Autodesk Inventor part; units mm, degrees
ref_plane "YZ Plane" through (0, 0, 0) normal (1, 0, 0) x (0, 1, 0)
ref_plane "XZ Plane" through (0, 0, 0) normal (0, 1, 0) x (-1, 0, 0)
ref_plane "XY Plane" through (0, 0, 0) normal (0, 0, 1) x (1, 0, 0)
sketch "スケッチ1" plane through (0, 0, 0) normal (0, 0, 1) x (1, 0, 0)
  line L0 (0, 55) -> (20, 55)
  line L1 (20, 55) -> (20, 0)
  line L2 (20, 0) -> (0, 0)
  line L3 (0, 0) -> (0, 55)
  dimension "d0" = 20
  dimension "d1" = 55
extrude "押し出し1" add sketch "スケッチ1" along normal blind 10
chamfer "面取り1" distance 7 angle 45 4 edges at (20, 27.5, 10) (0, 27.5, 10) (10, 55, 10) (10, 0, 10)
sketch "スケッチ2" plane through (0, 0, 0) normal (0, 0, -1) x (-1, 0, 0)
  line L0 (0, 0) -> (-20, 0)
  line L1 (0, 55) -> (0, 0)
  line L2 (-20, 55) -> (0, 55)
  line L3 (-20, 0) -> (-20, 55)
  circle A0 centre (-10, 41.25) radius 0.8
  circle A1 centre (-10, 13.75) radius 0.8
  circle A2 centre (-10, 27.5) radius 0.8
  point P0 (-10, 55)
  dimension "d7" = 1.6
  dimension "d8" = 1.6
  dimension "d9" = 1.6
  dimension "d10" = 13.75
  dimension "d11" = 13.75
  dimension "d12" = 13.75
  dimension "d13" = 13.75
extrude "押し出し2" cut sketch "スケッチ2" against normal through all contours A0 | A1 | A2
sketch "スケッチ3" plane through (0, 0, 10) normal (0, 0, 1) x (1, 0, 0)
  circle A0 centre (10, 41.25) radius 0.8
  circle A1 centre (10, 27.5) radius 0.8
  circle A2 centre (10, 13.75) radius 0.8
  circle A3 centre (10, 27.5) radius 0.8
  circle A4 centre (10, 41.25) radius 0.8
  line L0 (7, 7) -> (7, 48)
  line L1 (13, 7) -> (7, 7)
  line L2 (13, 48) -> (13, 7)
  line L3 (7, 48) -> (13, 48)
  circle A5 centre (10, 41.25) radius 2.5
  circle A6 centre (10, 27.5) radius 2.5
  circle A7 centre (10, 13.75) radius 2.5
  point P0 (0, 0)
  dimension "d16" = 5
  dimension "d17" = 5
  dimension "d18" = 5
extrude "押し出し3" cut sketch "スケッチ3" against normal blind 8.5 contours A5 | A6 | A7
equation "\"d10\" = d13"
equation "\"d11\" = d13"
equation "\"d12\" = d13"
properties part number "shield"
Read the model definition and answer for the solid it produces. Units are mm, in the model's axes. A direction names the side the tool comes from. Give positions to 0.01 mm unless a question says otherwise; leave off trailing zeros. Write each loop counter-clockwise with the first axis right and the second up, starting at its lowest first coordinate (ties: lowest second). Pieces come first, ordered by that corner, then holes. Notation, with made-up numbers: (-21, -27.5) -> (23, -27.5) arc R24 cw to (23, -13.5) -> close; hole circle Ø4 at (5.25, -11.75). An arc over 180 degrees is marked (long way). Answer as a JSON object with one key per item and string values. Group by question number.
1) Find section C-C (x = 10). Count the separate pieces of the cut face and the enclosed holes in it, and give its area (3 significant figures).
2) A tool of negligible diameter and unlimited length cuts with its end or side. For faces 4 (the flat face through (9, 14, 1.5)), 5 (the flat face through (10, 3, 6)), from which of +Z, -Z, +X, -X, +Y, -Y can it reach the whole face along a straight path? Write none if from no direction.
3) Find section A-A (y = 27.5). Write down the section's boundary in (x, z), and give its area (3 significant figures).
4) Find section D-D (x = 15.75). Write down the section's boundary in (y, z).
5) Find section B-B (z = 2.25). Write down the section's boundary in (x, y).
6) Consider L1, parallel to Y at x = 10, z = 0.9; L2, parallel to Y at x = 10, z = 5.5; L3, parallel to X at y = 27.5, z = 0.4. Determine where each line is inside the solid, lowest interval first. Write a range as from..to.
7) The mould has two halves that part along Y. Classify faces 1 (the flat face through (20, 28, 1)), 2 (the flat face through (10, 55, 1)), 3 (the cylindrical face through (10.104, 14.543, 0.74)): +Y half, -Y half, draft (parallel to the pull), parting line (faces both ways), or undercut.
8) Each of these flat-tipped pins is pushed along its axis until it touches: P1, Ø1.5, axis at x = 10, y = 40, coming from the +Z side; P2, Ø3, axis at x = 4, y = 30.5, coming from the +Z side. Where does it stop, or does it pass through?
Values follow:
{
 "1": {"separate pieces": "4", "enclosed holes": "0", "area": "366 mm2"},
 "2": {"face 4": "+Z", "face 5": "+Z, +X, -X, -Y"},
 "3": {"outline": "(0, 0) -> (9.2, 0) -> (9.2, 1.5) -> (7.5, 1.5) -> (7.5, 10) -> (7, 10) -> (0, 3) -> close; (10.8, 0) -> (20, 0) -> (20, 3) -> (13, 10) -> (12.5, 10) -> (12.5, 1.5) -> (10.8, 1.5) -> close", "area": "106 mm2"},
 "4": {"outline": "(0, 0) -> (55, 0) -> (55, 3) -> (50.75, 7.25) -> (4.25, 7.25) -> (0, 3) -> close"},
 "5": {"outline": "(0, 0) -> (20, 0) -> (20, 55) -> (0, 55) -> close; hole circle Ø5 at (10, 13.75); hole circle Ø5 at (10, 27.5); hole circle Ø5 at (10, 41.25)"},
 "6": {"L1": "y = 0..12.95, 14.55..26.7, 28.3..40.45, 42.05..55", "L2": "y = 2.5..11.25, 16.25..25, 30..38.75, 43.75..52.5", "L3": "x = 0..9.2, 10.8..20"},
 "7": {"face 1": "draft", "face 2": "+Y half", "face 3": "undercut"},
 "8": {"P1": "stops at z = 1.5", "P2": "stops at z = 8.5"}
}
